from build123d import *

# Parameters (mm, degrees)
BOSS_EXTRUDE1_DEPTH = 2
BOSS_EXTRUDE2_DEPTH = 5
SKETCH4_W           = 51.8
SKETCH4_H           = 8.22
SKETCH4_H_2         = 5.68
CUT_EXTRUDE1_DEPTH  = 2
BOSS_EXTRUDE3_DEPTH = 5
SKETCH8_W           = 5.977250124
SKETCH8_H           = 14
CUT_EXTRUDE3_DEPTH  = 4
SKETCH9_W           = 9.791789178
SKETCH9_H           = 32.4
CUT_EXTRUDE4_DEPTH  = 4


with BuildPart() as part:
    # Sketch2 → Boss-Extrude1 (new body)
    with BuildSketch(Plane(origin=(0, 0, 0), x_dir=(1, 0, 0), z_dir=(0, 1, 0))):
        with BuildLine():
            Line((-29.941284627, -27.87), (30.48, -27.87))
            ThreePointArc((30.48, -27.87), (34.050723427, -26.374261545), (35.489363684, -22.780153375))
            ThreePointArc((35.489363684, -22.780153375), (34.068, 0), (35.489363684, 22.780153375))
            ThreePointArc((35.489363684, 22.780153375), (34.050723427, 26.374261545), (30.48, 27.87))
            Line((30.48, 27.87), (-29.941284627, 27.87))
            ThreePointArc((-29.941284627, 27.87), (-33.058077828, 26.779680312), (-34.815550633, 23.984240056))
            ThreePointArc((-34.815550633, 23.984240056), (-37.522, 0), (-34.815550633, -23.984240056))
            ThreePointArc((-34.815550633, -23.984240056), (-33.058077828, -26.779680312), (-29.941284627, -27.87))
        make_face()
    extrude(amount=BOSS_EXTRUDE1_DEPTH)

    # Sketch3 → Boss-Extrude2 (add)
    with BuildSketch(Plane.XZ):
        with BuildLine():
            Line((-29.941284627, -26.67), (30.48, -26.67))
            ThreePointArc((30.48, -26.67), (33.174076836, -25.554076836), (34.29, -22.86))
            ThreePointArc((34.29, -22.86), (32.868, 0), (34.29, 22.86))
            ThreePointArc((34.29, 22.86), (33.174076836, 25.554076836), (30.48, 26.67))
            Line((30.48, 26.67), (-29.941284627, 26.67))
            ThreePointArc((-29.941284627, 26.67), (-32.31004746, 25.841357037), (-33.645726791, 23.716822443))
            ThreePointArc((-33.645726791, 23.716822443), (-36.322, 0), (-33.645726791, -23.716822443))
            ThreePointArc((-33.645726791, -23.716822443), (-32.31004746, -25.841357037), (-29.941284627, -26.67))
        make_face()
        with BuildLine():
            Line((30.48, 25.67), (-29.941284627, 25.67))
            ThreePointArc((-29.941284627, 25.67), (-31.686688819, 25.059420975), (-32.67087359, 23.493974431))
            ThreePointArc((-32.67087359, 23.493974431), (-35.322, 0), (-32.67087359, -23.493974431))
            ThreePointArc((-32.67087359, -23.493974431), (-31.686688819, -25.059420975), (-29.941284627, -25.67))
            Line((-29.941284627, -25.67), (30.48, -25.67))
            ThreePointArc((30.48, -25.67), (32.446567575, -24.867165158), (33.289413465, -22.917410657))
            ThreePointArc((33.289413465, -22.917410657), (31.868, 0), (33.289413465, 22.917410657))
            ThreePointArc((33.289413465, 22.917410657), (32.446567575, 24.867165158), (30.48, 25.67))
        make_face(mode=Mode.SUBTRACT)
    extrude(amount=BOSS_EXTRUDE2_DEPTH)

    # Sketch4 → Cut-Extrude1 (cut)
    with BuildSketch(Plane(origin=(0, 2, 0), x_dir=(1, 0, 0), z_dir=(0, 1, 0))):
        with Locations((-0.000636316, 21.56)):
            Rectangle(SKETCH4_W, SKETCH4_H)
        with Locations((-0.000636316, -22.83)):
            Rectangle(SKETCH4_W, SKETCH4_H_2)
    extrude(amount=-CUT_EXTRUDE1_DEPTH, mode=Mode.SUBTRACT)

    # Sketch6 → Boss-Extrude3 (add)
    with BuildSketch(Plane.XZ):
        with BuildLine():
            Line((-36.326051564, 16), (-34.100805436, 16))
            ThreePointArc((-34.100805436, 16), (-35.322, 0), (-34.100805436, -16))
            Line((-34.100805436, -16), (-36.326051564, -16))
            ThreePointArc((-36.326051564, -16), (-37.522, 0), (-36.326051564, 16))
        make_face()
    extrude(amount=BOSS_EXTRUDE3_DEPTH)

    # Sketch8 → Cut-Extrude3 (cut)
    with BuildSketch(Plane.XZ.offset(5)):
        with Locations((32.449466872, 0)):
            Rectangle(SKETCH8_W, SKETCH8_H)
    extrude(amount=-CUT_EXTRUDE3_DEPTH, mode=Mode.SUBTRACT)

    # Sketch9 → Cut-Extrude4 (cut)
    with BuildSketch(Plane(origin=(0, -5, 0), x_dir=(-1, 0, 0), z_dir=(0, -1, 0))):
        with Locations((35.349982691, 0)):
            Rectangle(SKETCH9_W, SKETCH9_H)
    extrude(amount=-CUT_EXTRUDE4_DEPTH, mode=Mode.SUBTRACT)


solid = part.part
Source: CAD feature listing. Evaluate the final solid. Frame: model axes, mm. A direction names the side the tool comes from. Round coordinates to 2 decimals unless told otherwise and drop trailing zeros. Loops run counter-clockwise (first coordinate to the right, second up) from the corner with the lowest first, then second, coordinate; pieces in that order, holes last. Notation, with made-up numbers: M 48,-13 L 75,-13 A11 cw 75,-2 Z; hole C 57.5,-10.75 d3. An arc over 180 degrees is marked long. Answer as CSV lines item,"result".
Q1. Reachability of faces 1 (the face through (33.144, -2.465, -25.584)), 2 (the face through (0, 1, 19.99)), 3 (the face through (33.204, -2.465, 25.524)) from +Z, -Z, +X, -X, +Y, -Y: full face, straight path, thin tool, end or side. Return the list, or none.
Verdict:
face 1,"-Z, +X, -Y"
face 2,"+Y, -Y"
face 3,"+Z, +X, -Y"
Q2. Cut plane B-B (x = -4.5). Return the cut outline in (y, z).
Verdict:
outline,"M -5,-26.67 L 0,-26.67 L 0,-27.87 L 2,-27.87 L 2,-25.67 L -5,-25.67 Z; M -5,25.67 L 2,25.67 L 2,27.87 L 0,27.87 L 0,26.67 L -5,26.67 Z; M 0,-17.45 L 2,-17.45 L 2,19.99 L 0,19.99 Z"
Q3. Cut plane D-D (x = 29.5). Return the cut outline in (y, z), plus the area to 3 significant figures.
Verdict:
outline,"M -5,-26.67 L 0,-26.67 L 0,-27.87 L 2,-27.87 L 2,27.87 L 0,27.87 L 0,26.67 L -5,26.67 L -5,25.67 L 0,25.67 L 0,-25.67 L -5,-25.67 Z"
area,"121 mm^2"
Q4. Line query: line 1 along Z through (x, y) = (-21.5, 0.25); line 2 along Z through (x, y) = (-24, -3.5); line 3 along Y through (x, z) = (25, 0.5). Output: solid intervals per line, ascending.
Verdict:
line 1,"z = -27.87 to -25.67, -17.45 to 19.99, 25.67 to 27.87"
line 2,"z = -26.67 to -25.67, 25.67 to 26.67"
line 3,"y = 0 to 2"
Q5. Cut plane C-C (y = 1.25). Return the cut outline in (x, z).
Verdict:
outline,"M -34.82,-23.98 A5 ccw -29.94,-27.87 L 30.48,-27.87 A5.01 ccw 35.49,-22.78 A183.26 cw 35.49,22.78 A5.01 ccw 30.48,27.87 L -29.94,27.87 A5 ccw -34.82,23.98 A107.63 ccw Z; hole M -25.9,-25.67 L 25.9,-25.67 L 25.9,-17.45 L -25.9,-17.45 Z; hole M -25.9,19.99 L 25.9,19.99 L 25.9,25.67 L -25.9,25.67 Z"
Q6. Contact query for flat-ended pins moving along their axis: pin 1 (10 mm diameter, centred on x = 2.5, z = 11, fed in from -Y); pin 2 (3 mm diameter, centred on x = -22.5, y = -3, fed in from +Z); pin 3 (1.2 mm diameter, centred on x = 32.5, z = 1, fed in from -Y). Output: stop coordinate, or through.
Verdict:
pin 1,"stops at y = 0"
pin 2,"stops at z = 26.67"
pin 3,"stops at y = -1"
Q7. Cut plane A-A (y = -4). Return the cut outline in (x, z).
Verdict:
outline,"M -35.08,-16.2 A106.43 ccw -33.65,-23.72 A3.8 ccw -29.94,-26.67 L 30.48,-26.67 A3.81 ccw 34.29,-22.86 A184.46 cw 33,-7 L 32,-7 A185.46 ccw 33.29,-22.92 A2.81 cw 30.48,-25.67 L -29.94,-25.67 A2.8 cw -32.67,-23.49 A105.43 cw -34.07,-16.2 Z; M -35.08,16.2 L -34.07,16.2 A105.43 cw -32.67,23.49 A2.8 cw -29.94,25.67 L 30.48,25.67 A2.81 cw 33.29,22.92 A185.46 ccw 32,7 L 33,7 A184.46 cw 34.29,22.86 A3.81 ccw 30.48,26.67 L -29.94,26.67 A3.8 ccw -33.65,23.72 A106.43 ccw Z"
Q8. Pull-direction query (Y, two-part tool) for faces 4 (the face through (-2, 2, 0)), 5 (the face through (32.468, -2.465, 24.846)), 6 (the face through (-1, 0, 0)); classes: +Y half, -Y half, draft (parallel to the pull), parting line (faces both ways), or undercut.
Verdict:
face 4,"+Y half"
face 5,"draft"
face 6,"-Y half"
